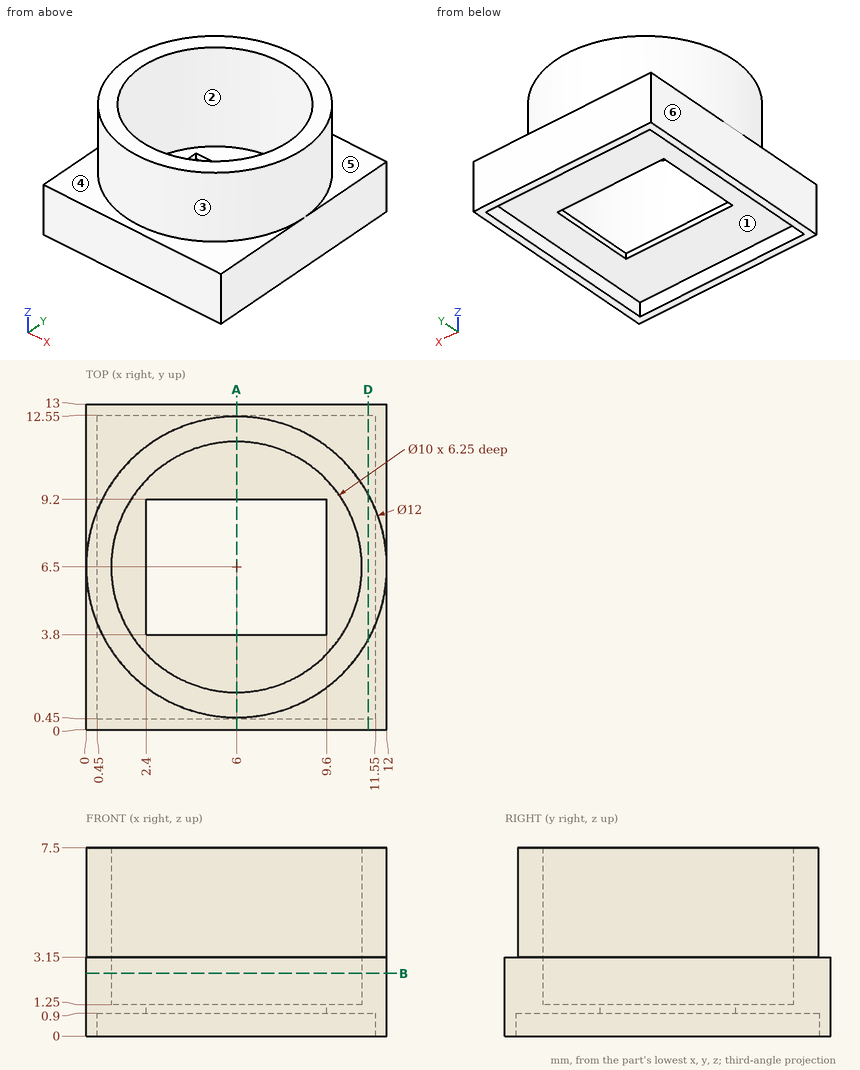
Job drawing, mm, ordinate dimensions from the low corner. One solid piece. A direction names the side the tool comes from. Round coordinates to 2 decimals unless told otherwise and drop trailing zeros. Order: outer loops, then holes, each group sorted by start corner. A loop starts at its lowest first (then second) coordinate and runs counter-clockwise, first axis right, second up. Notation, with made-up numbers: (72, 32.25) - (89, 32.25) arc R18 cw to (89, 49.25) - close; hole circle Ø3 at (84, 66). An arc over 180 degrees is marked (long way). Use CSV: the item, a comma, the result in double quotes. Start each with the question number.
1) Saw through at D-D (x = 11.25). List the corners of the cut face in (y, z), and give its area (3 significant figures).
2) Saw through at B-B (z = 2.5). List the corners of the cut face in (x, y).
3) Tool access for the marked faces 5 and 6: list every direction of +Z, -Z, +X, -X, +Y, -Y with a clear straight run to the whole face (end or side of a thin tool).
4) Two-plate mould, pull along X, no slides. Class the marked faces 1, 2, 3 and 4: pulls with the +X half, pulls with the -X half, needs draft (parallel to the pull), parting line crosses it, or undercut.
5) Saw through at A-A (x = 6). List the corners of the cut face in (y, z), and give its area (3 significant figures).
6) Wall check: L1, parallel to Y at x = 6, z = 3.25; L2, parallel to Y at x = 6, z = 2.75; L3, parallel to Z at x = 11, y = 4.25. Give the ranges that are in metal, low to high. Write a range as [from, to].
7) Pin check, flat tips, straight feed: pin 1 Ø3 at (x, y) = (6, 8.5) entering from +Z; pin 2 Ø1 at (y, z) = (2, 5.5) entering from +X; pin 3 Ø1 at (x, y) = (10.5, 2.5) entering from -Z. Stop position of each tip, or through.
Values follow:
1,outline,"(0, 0) - (0.45, 0) - (0.45, 0.9) - (12.55, 0.9) - (12.55, 0) - (13, 0) - (13, 3.15) - (9.4, 3.15) - (9.4, 7.5) - (3.6, 7.5) - (3.6, 3.15) - (0, 3.15) - close"
1,area,"55.3 mm2"
2,outline,"(0, 0) - (12, 0) - (12, 13) - (0, 13) - close; hole circle Ø10 at (6, 6.5)"
3,face 5,"+Z, +Y"
3,face 6,"+Z, -Z, -X, +Y, -Y"
4,face 1,"undercut"
4,face 2,"undercut"
4,face 3,"parting line crosses it"
4,face 4,"needs draft"
5,outline,"(0, 0) - (0.45, 0) - (0.45, 0.9) - (3.8, 0.9) - (3.8, 1.25) - (1.5, 1.25) - (1.5, 7.5) - (0.5, 7.5) - (0.5, 3.15) - (0, 3.15) - close; (9.2, 0.9) - (12.55, 0.9) - (12.55, 0) - (13, 0) - (13, 3.15) - (12.5, 3.15) - (12.5, 7.5) - (11.5, 7.5) - (11.5, 1.25) - (9.2, 1.25) - close"
5,area,"17.9 mm2"
6,L1,"y = [0.5, 1.5], [11.5, 12.5]"
6,L2,"y = [0, 1.5], [11.5, 13]"
6,L3,"z = [0.9, 7.5]"
7,pin 1,"stops at z = 1.25"
7,pin 2,"stops at x = 10.47"
7,pin 3,"stops at z = 0.9"
